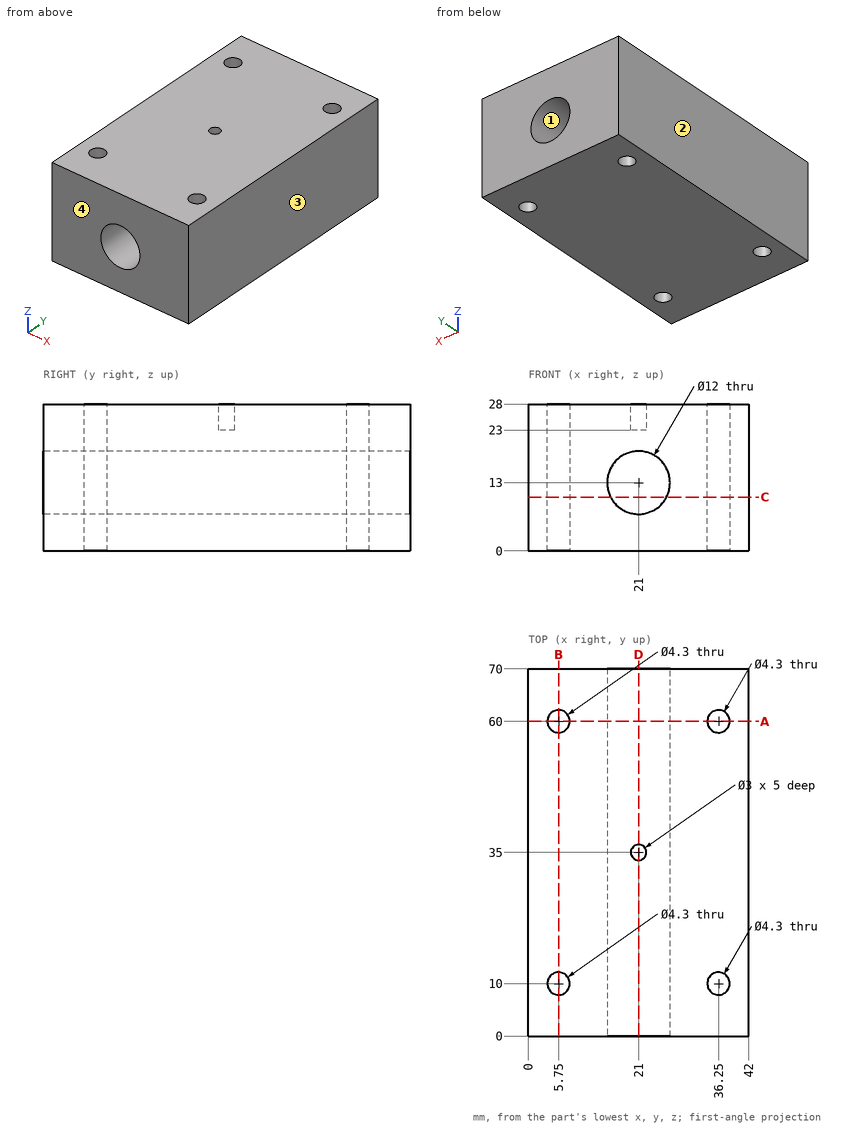
Here's the drawing with two shaded views (mm, measured from the low corner). I have some questions. Give positions to 0.01 mm unless a question says otherwise; leave off trailing zeros. Order: outer loops, then holes, each group sorted by start corner. A loop starts at its lowest first (then second) coordinate and runs counter-clockwise, first axis right, second up.
Q1. Suppose I cut it at A-A, the plane y = 60. Write out the boundary of the cut face in (x, z), and give its area (3 significant figures).
Q2. Suppose I cut it at B-B, the plane x = 5.75. Write out the boundary of the cut face in (y, z), and give its area (3 significant figures).
Q3. Suppose I cut it at D-D, the plane x = 21. Write out the boundary of the cut face in (y, z), and give its area (4 significant figures).
Q4. We'd pull the mould along X, two halves only. Please class the marked faces 1, 2, 3 and 4: +X half, -X half, draft (parallel to the pull), parting line (faces both ways), or undercut.
Q5. Suppose I cut it at C-C, the plane z = 10.25. Write out the boundary of the cut face in (x, y).
Q6. If I drill on line 1 along Y through (x, z) = (5.75, 17.5); line 2 along Y through (x, z) = (5, 6.5); line 3 along Y through (x, z) = (21, 24.5), over which ranges is the centre line in solid material (lowest first)?
Q7. I'm going to push a flat-ended pin straight in: P1, Ø2.5, axis at x = 36.25, y = 10, coming from the +Z side. Where does the tip first touch, or does it pass through?
Solution:
1. outline: (0, 0) - (3.6, 0) - (3.6, 28) - (0, 28) - close; (7.9, 0) - (34.1, 0) - (34.1, 28) - (7.9, 28) - close; (38.4, 0) - (42, 0) - (42, 28) - (38.4, 28) - close; hole circle Ø12 at (21, 13)
1. area: 822 mm2
2. outline: (0, 0) - (7.85, 0) - (7.85, 28) - (0, 28) - close; (12.15, 0) - (57.85, 0) - (57.85, 28) - (12.15, 28) - close; (62.15, 0) - (70, 0) - (70, 28) - (62.15, 28) - close
2. area: 1,720 mm2
3. outline: (0, 0) - (70, 0) - (70, 7) - (0, 7) - close; (0, 19) - (70, 19) - (70, 28) - (36.5, 28) - (36.5, 23) - (33.5, 23) - (33.5, 28) - (0, 28) - close
3. area: 1,105 mm2
4. face 1: undercut
4. face 2: -X half
4. face 3: +X half
4. face 4: draft
5. outline: (0, 0) - (15.67, 0) - (15.67, 70) - (0, 70) - close; (26.33, 0) - (42, 0) - (42, 70) - (26.33, 70) - close; hole circle Ø4.3 at (5.75, 10); hole circle Ø4.3 at (5.75, 60); hole circle Ø4.3 at (36.25, 10); hole circle Ø4.3 at (36.25, 60)
6. line 1: y = 0 to 7.85, 12.15 to 57.85, 62.15 to 70
6. line 2: y = 0 to 7.99, 12.01 to 57.99, 62.01 to 70
6. line 3: y = 0 to 33.5, 36.5 to 70
7. P1: passes through
